from build123d import *

# Parameters (mm, degrees)
SKETCH1_W                 = 45.2
SKETCH1_H                 = 24.6
BOSS_EXTRUDE1_DEPTH       = 35.8
BOSS_EXTRUDE2_DEPTH       = 4.5
SKETCH4_R                 = 1.4
CUT_EXTRUDE1_DEPTH        = 68.568483778
LPATTERN1_COUNT           = 3
LPATTERN1_PITCH           = 17.5
LPATTERN1_COUNT_DIR2      = 2
LPATTERN1_PITCH_DIR2      = 30
SKETCH6_R                 = 1.4
CUT_EXTRUDE2_DEPTH        = 68.568483778
LPATTERN2_COUNT           = 2
LPATTERN2_PITCH           = 28.5
LPATTERN2_COPY_1_SKETCH_R = 1.4
LPATTERN2_COPY_1_DEPTH    = 68.568483778
LPATTERN2_COPY_2_SKETCH_R = 1.4
LPATTERN2_COPY_2_DEPTH    = 68.568483778
LPATTERN2_COPY_3_SKETCH_R = 1.4
LPATTERN2_COPY_3_DEPTH    = 68.568483778
LPATTERN2_COPY_4_SKETCH_R = 1.4
LPATTERN2_COPY_4_DEPTH    = 68.568483778
LPATTERN2_COPY_5_SKETCH_R = 1.4
LPATTERN2_COPY_5_DEPTH    = 68.568483778


with BuildPart() as part:
    # Sketch1 → Boss-Extrude1 (new body)
    with BuildSketch(Plane.XY):
        with Locations((22.6, 12.3)):
            Rectangle(SKETCH1_W, SKETCH1_H)
    extrude(amount=BOSS_EXTRUDE1_DEPTH)

    # Sketch3 → Boss-Extrude2 (add)
    with BuildSketch(Plane.XY.offset(33)):
        Polygon((0, 24.6), (6.26496063, 30.1), (44.26496063, 30.1), (50.7, 24.8), (50.7, -0.2), (44.26496063, -5.5), (6.26496063, -5.5), (0, 0), (45.2, 0), (45.2, 24.6), align=None)
    boss_extrude2 = extrude(amount=-BOSS_EXTRUDE2_DEPTH)

    # Sketch4 → Cut-Extrude1 (cut, through all)
    with BuildSketch(Plane.XY.offset(33)):
        with Locations((6.7, 27.1)):
            Circle(SKETCH4_R)
    cut_extrude1 = extrude(amount=-CUT_EXTRUDE1_DEPTH, mode=Mode.SUBTRACT)

    # LPattern1: Cut-Extrude1 3 × 2
    with Locations(*[(i * LPATTERN1_PITCH, -j * LPATTERN1_PITCH_DIR2, 0) for i in range(LPATTERN1_COUNT) for j in range(LPATTERN1_COUNT_DIR2) if (i, j) != (0, 0)]):
        add(cut_extrude1, mode=Mode.SUBTRACT)

    # Sketch6 → Cut-Extrude2 (cut, through all)
    with BuildSketch(Plane.XY.offset(33)):
        with Locations((47.7, 20.5)):
            Circle(SKETCH6_R)
        with Locations((47.7, 3.1)):
            Circle(SKETCH6_R)
    cut_extrude2 = extrude(amount=-CUT_EXTRUDE2_DEPTH, mode=Mode.SUBTRACT)

    # LPattern2: Boss-Extrude2, Cut-Extrude1, Cut-Extrude2 ×2
    with Locations(*[(0, 0, -i * LPATTERN2_PITCH) for i in range(1, LPATTERN2_COUNT)]):
        add(boss_extrude2)
        add(cut_extrude1, mode=Mode.SUBTRACT)
        add(cut_extrude2, mode=Mode.SUBTRACT)

    # LPattern2 copy 1 sketch → LPattern2 copy 1 (cut, through all)
    with BuildSketch(Plane(origin=(0, -30, 4.5), x_dir=(1, 0, 0), z_dir=(0, 0, 1))):
        with Locations((6.7, 27.1)):
            Circle(LPATTERN2_COPY_1_SKETCH_R)
    extrude(amount=-LPATTERN2_COPY_1_DEPTH, mode=Mode.SUBTRACT)

    # LPattern2 copy 2 sketch → LPattern2 copy 2 (cut, through all)
    with BuildSketch(Plane(origin=(17.5, 0, 4.5), x_dir=(1, 0, 0), z_dir=(0, 0, 1))):
        with Locations((6.7, 27.1)):
            Circle(LPATTERN2_COPY_2_SKETCH_R)
    extrude(amount=-LPATTERN2_COPY_2_DEPTH, mode=Mode.SUBTRACT)

    # LPattern2 copy 3 sketch → LPattern2 copy 3 (cut, through all)
    with BuildSketch(Plane(origin=(17.5, -30, 4.5), x_dir=(1, 0, 0), z_dir=(0, 0, 1))):
        with Locations((6.7, 27.1)):
            Circle(LPATTERN2_COPY_3_SKETCH_R)
    extrude(amount=-LPATTERN2_COPY_3_DEPTH, mode=Mode.SUBTRACT)

    # LPattern2 copy 4 sketch → LPattern2 copy 4 (cut, through all)
    with BuildSketch(Plane(origin=(35, 0, 4.5), x_dir=(1, 0, 0), z_dir=(0, 0, 1))):
        with Locations((6.7, 27.1)):
            Circle(LPATTERN2_COPY_4_SKETCH_R)
    extrude(amount=-LPATTERN2_COPY_4_DEPTH, mode=Mode.SUBTRACT)

    # LPattern2 copy 5 sketch → LPattern2 copy 5 (cut, through all)
    with BuildSketch(Plane(origin=(35, -30, 4.5), x_dir=(1, 0, 0), z_dir=(0, 0, 1))):
        with Locations((6.7, 27.1)):
            Circle(LPATTERN2_COPY_5_SKETCH_R)
    extrude(amount=-LPATTERN2_COPY_5_DEPTH, mode=Mode.SUBTRACT)


solid = part.part
For this review, take the finished solid that the model builds, in its own axes (mm). A direction names the side the tool comes from. Give positions to 0.01 mm unless a question says otherwise; leave off trailing zeros. Loops run counter-clockwise (first coordinate to the right, second up) from the corner with the lowest first, then second, coordinate; pieces in that order, holes last.
Item 1: Take a section at C-C, the plane x = 47.7. State the section outline as (y, z) points.
Item 2: Take a section at A-A, the plane z = 3.5. Give the number of separate pieces and of enclosed holes in the cut face, and give its area (3 significant figures).
Item 3: Take a section at B-B, the plane y = 3.1. State the section outline as (x, z) points.
Item 4: Insertion check: pin 1 (4 mm diameter, centred on x = 8, z = 14.5, fed in from -Y); pin 2 (1.7 mm diameter, centred on x = 47.7, y = 20.5, fed in from -Z); pin 3 (3.5 mm diameter, centred on x = 24.2, y = -2.9, fed in from +Z); pin 4 (1.4 mm diameter, centred on y = 10, z = 34.5, fed in from +X). Each pin has a flat end and moves straight along its axis. Give the tip position at first contact, or say it passes through.
Item 5: Draft analysis for pull direction Y (two halves, no side actions). For faces 4 (the flat face through (22, 24.6, 34)), 5 (the cylindrical face through (40.3, 27.16, 2.28)), 6 (the cylindrical face through (46.3, 3.16, 2.28)), 7 (the flat face through (45.2, 12, 16)), state which applies: +Y half, -Y half, draft (parallel to the pull), parting line (faces both ways), or undercut.
Item 6: For line 1 along Y through (x, z) = (41.7, 31.6); line 2 along X through (y, z) = (3, 1); line 3 along X through (y, z) = (27, 31), list the stretches that pass through material, from the lowest coordinate up.
Item 7: Tool access review of faces 1 (the flat face through (33, -1, 4.5)), 2 (the flat face through (45.2, 12, 34)), 3 (the flat face through (22, 0, 34)): name each direction out of +Z, -Z, +X, -X, +Y, -Y from which nothing blocks a thin tool from reaching the whole face with its end or side.
Calculated:
1. outline: (-2.67, 0) - (1.7, 0) - (1.7, 4.5) - (-2.67, 4.5) - close; (-2.67, 28.5) - (1.7, 28.5) - (1.7, 33) - (-2.67, 33) - close; (4.5, 0) - (19.1, 0) - (19.1, 4.5) - (4.5, 4.5) - close; (4.5, 28.5) - (19.1, 28.5) - (19.1, 33) - (4.5, 33) - close; (21.9, 0) - (27.27, 0) - (27.27, 4.5) - (21.9, 4.5) - close; (21.9, 28.5) - (27.27, 28.5) - (27.27, 33) - (21.9, 33) - close
2. separate pieces: 1
2. enclosed holes: 8
2. area: 1,690 mm2
3. outline: (0, 0) - (46.3, 0) - (46.3, 4.5) - (45.2, 4.5) - (45.2, 28.5) - (46.3, 28.5) - (46.3, 33) - (45.2, 33) - (45.2, 35.8) - (0, 35.8) - close; (49.1, 0) - (50.7, 0) - (50.7, 4.5) - (49.1, 4.5) - close; (49.1, 28.5) - (50.7, 28.5) - (50.7, 33) - (49.1, 33) - close
4. pin 1: stops at y = 0
4. pin 2: passes through
4. pin 3: stops at z = 33
4. pin 4: stops at x = 45.2
5. face 4: +Y half
5. face 5: undercut
5. face 6: undercut
5. face 7: draft
6. line 1: y = -5.5 to -4.3, -1.5 to 25.7, 28.5 to 30.1
6. line 2: x = 0 to 46.3, 49.1 to 50.7
6. line 3: x = 2.73 to 5.3, 8.1 to 22.8, 25.6 to 40.3, 43.1 to 48.03
7. face 1: +X
7. face 2: +Z, +X, +Y, -Y
7. face 3: +Z, +X, -X, -Y
